Read the model definition and answer for the solid it produces. Units are mm, in the model's axes. Face numbers are marked on the shaded views. Round coordinates to 2 decimals unless told otherwise and drop trailing zeros. Order: outer loops, then holes, each group sorted by start corner. A loop starts at its lowest first (then second) coordinate and runs counter-clockwise, first axis right, second up. Notation, with made-up numbers: (78.5, -1) -> (95.5, -1) arc R33 ccw to (95.5, 35) -> close; hole circle Ø8 at (-20, 85.5). An arc over 180 degrees is marked (long way). One line per item, written item: value. Start each with the question number.
1. Section D-D (y = -4.75) is taken. Give the vertices of the cut face in (x, z).
2. Flat-ended cylindrical pins translate along their axes: pin 1 Ø4 at (y, z) = (-11.5, 32) entering from -X; pin 2 Ø6 at (y, z) = (-4.5, 74) entering from -X; pin 3 Ø1 at (y, z) = (-22.5, 89) entering from -X; pin 4 Ø3 at (x, y) = (25.5, -13.5) entering from +Z. Find the tip coordinate at first contact, or state that the pin passes through.
3. Section B-B (z = 85) is taken. Give the vertices of the cut face in (x, y), then the cut area to 3 significant figures.
4. The mould has two halves that part along X. Classify the marked faces 1, 2, 3 and 4: released by +X, released by -X, zero draft, split by the parting line, or undercut.
5. Section A-A (y = -19) is taken. Give the vertices of the cut face in (x, z).
6. Section C-C (x = -49) is taken. Give the vertices of the cut face in (y, z).
7. Consider line 1 (X direction, y = -5.5, z = 76.2); line 2 (X direction, y = -20.75, z = 32); line 3 (X direction, y = -15, z = 91). Determine where each line is inside the solid, lowest interval first.
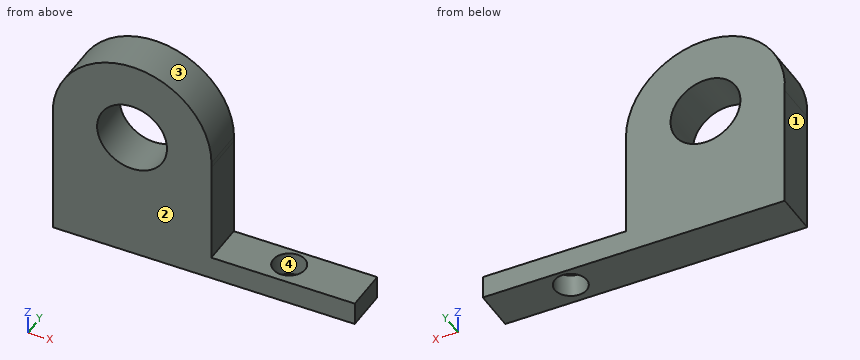
from build123d import *

# Parameters (mm, degrees)
F0_W     = 84.456712
F0_H     = 13.497178
F1_DEPTH = 25.4
F2_R     = 9.965613
F3_DEPTH = 25.4
F4_R     = 9.424237
F5_DEPTH = 25.4


with BuildPart() as f1:
    # F0 (on Front) → F1 (new body)
    with BuildSketch(Plane.XZ):
        with BuildLine():
            ThreePointArc((0.107788, 76.2), (-48.259449, 122.952477), (-93.343288, 73.026219))
            Line((-93.343288, 73.026219), (-93.343288, 76.2))
            Line((-93.343288, 76.2), (-67.245644, 76.2))
            ThreePointArc((-67.245644, 76.2), (-46.671644, 96.774), (-26.097644, 76.2))
            Line((-26.097644, 76.2), (0, 76.2))
            Line((0, 76.2), (0, 73.026219))
            ThreePointArc((0, 73.026219), (0.080833, 74.612195), (0.107788, 76.2))
        make_face()
        with BuildLine():
            Line((-93.343288, 76.2), (-93.343288, 73.026219))
            ThreePointArc((-93.343288, 73.026219), (-46.671644, 29.420568), (0, 73.026219))
            Line((0, 73.026219), (0, 76.2))
            Line((0, 76.2), (-26.097644, 76.2))
            ThreePointArc((-26.097644, 76.2), (-46.671644, 55.626), (-67.245644, 76.2))
            Line((-67.245644, 76.2), (-93.343288, 76.2))
        make_face()
        with BuildLine():
            Line((-93.343288, 73.026219), (-93.343288, 0))
            Line((-93.343288, 0), (0, 0))
            Line((0, 0), (0, 13.497178))
            Line((0, 13.497178), (0, 73.026219))
            ThreePointArc((0, 73.026219), (-46.671644, 29.420568), (-93.343288, 73.026219))
        make_face()
        with Locations((42.228356, 6.748589)):
            Rectangle(F0_W, F0_H)
    extrude(amount=F1_DEPTH)

    # F2 (on Top) → F3 (cut)
    with BuildSketch(Plane.XY):
        with Locations((45.747578, -12.0396)):
            Circle(F2_R)
    extrude(amount=-F3_DEPTH, mode=Mode.SUBTRACT)

    # F4 (on face) → F5 (cut)
    with BuildSketch(Plane.XY.offset(13.497178)):
        with Locations((38.751498, -11.754938)):
            Circle(F4_R)
    extrude(amount=-F5_DEPTH, mode=Mode.SUBTRACT)


solid = f1.part
Answer:
1. outline: (-93.34, 0) -> (32.45, 0) -> (32.45, 13.5) -> (0, 13.5) -> (0, 73.03) arc R46.78 ccw to (0.11, 76.2) arc R46.78 ccw (long way) to (-93.34, 73.03) -> close; (45.06, 0) -> (84.46, 0) -> (84.46, 13.5) -> (45.06, 13.5) -> close; hole circle Ø41.15 at (-46.67, 76.2)
2. pin 1: x = -93.34
2. pin 2: x = -93.45
2. pin 3: x = -91.81
2. pin 4: z = 13.5
3. outline: (-92.62, -25.4) -> (-65.27, -25.4) -> (-65.27, 0) -> (-92.62, 0) -> close; (-28.07, -25.4) -> (-0.73, -25.4) -> (-0.73, 0) -> (-28.07, 0) -> close
3. area: 1,390 mm^2
4. face 1: released by -X
4. face 2: zero draft
4. face 3: split by the parting line
4. face 4: undercut
5. outline: (-93.34, 0) -> (32.72, 0) -> (32.72, 13.5) -> (0, 13.5) -> (0, 73.03) arc R46.78 ccw to (0.11, 76.2) arc R46.78 ccw (long way) to (-93.34, 73.03) -> close; (44.78, 0) -> (84.46, 0) -> (84.46, 13.5) -> (44.78, 13.5) -> close; hole circle Ø41.15 at (-46.67, 76.2)
6. outline: (-25.4, 0) -> (0, 0) -> (0, 55.76) -> (-25.4, 55.76) -> close; (-25.4, 96.64) -> (0, 96.64) -> (0, 122.92) -> (-25.4, 122.92) -> close
7. line 1: -93.45 to -67.25, -26.1 to 0.11
7. line 2: -93.34 to 0
7. line 3: -91.05 to -60.96, -32.38 to -2.3
